from build123d import *

# Parameters (mm, degrees)
SKETCH1_R           = 1.75
SKETCH1_R_2         = 3.175
SKETCH1_R_3         = 1.778
BOSS_EXTRUDE1_DEPTH = 5.461


with BuildPart() as part:
    # Sketch1 → Boss-Extrude1 (new body)
    with BuildSketch(Plane(origin=(0, 0, 0), x_dir=(1, 0, 0), z_dir=(0, 1, 0))):
        with BuildLine():
            Line((-36.075553112, 16.34222836), (-43.713289862, 9.687095487))
            ThreePointArc((-43.713289862, 9.687095487), (-46.071262537, 8.895051227), (-48.298660873, 10.002329828))
            Line((-48.298660873, 10.002329828), (-49.01441114, 10.823757773))
            ThreePointArc((-49.01441114, 10.823757773), (-49.677098428, 12.125807852), (-49.646194202, 13.586469955))
            ThreePointArc((-49.646194202, 13.586469955), (-47.370124011, 20.134748964), (-44.234733225, 26.317772344))
            ThreePointArc((-44.234733225, 26.317772344), (-39.855484626, 29.811728531), (-34.259632886, 29.543416329))
            Line((-34.259632886, 29.543416329), (5.363638877, 12.388760148))
            ThreePointArc((5.363638877, 12.388760148), (7.44200849, -11.263503435), (-13.499793526, -0.074664302))
            Line((-13.499793526, -0.074664302), (-36.075553112, 16.34222836))
        make_face()
        with Locations((8, 0)):
            Circle(SKETCH1_R, mode=Mode.SUBTRACT)
        with Locations((0, -8)):
            Circle(SKETCH1_R, mode=Mode.SUBTRACT)
        with Locations((-8, 0)):
            Circle(SKETCH1_R, mode=Mode.SUBTRACT)
        with Locations((0, 8)):
            Circle(SKETCH1_R, mode=Mode.SUBTRACT)
        Circle(SKETCH1_R_2, mode=Mode.SUBTRACT)
        with Locations((-20.862458922, 15.093717491)):
            Circle(SKETCH1_R_3, mode=Mode.SUBTRACT)
        with Locations((-37.413253893, 22.259284205)):
            Circle(SKETCH1_R_3, mode=Mode.SUBTRACT)
    extrude(amount=BOSS_EXTRUDE1_DEPTH)


solid = part.part
Geometry: final body of the model. Coordinates: model frame, mm. A direction names the side the tool comes from. Give positions to 0.01 mm unless a question says otherwise; leave off trailing zeros. Loops run counter-clockwise (first coordinate to the right, second up) from the corner with the lowest first, then second, coordinate; pieces in that order, holes last. Notation, with made-up numbers: (23, 4.5) - (42, 4.5) arc R10 ccw to (42, 17.5) - close; hole circle Ø4 at (-15.75, -12.75). An arc over 180 degrees is marked (long way). Answer as CSV lines item,"result". Start each with the question number.
1. Draft query along Z for faces 3 (the face through (-39.932, 2.692, -29.787)), 4 (the face through (-0.69, 2.69, 3.1)), 5 (the face through (-18, 5.461, -9)). Return one class per face: released by +Z, released by -Z, zero draft, split by the parting line, or undercut.
2. Section D-D, the plane y = 3.95. Give the number of separate pieces and of enclosed holes in the cut face, plus the area to 3 significant figures.
3. Reachability of faces 1 (the face through (-0.228, 2.692, -9.735)), 2 (the face through (-24.63, 2.69, -8.02)) from +Z, -Z, +X, -X, +Y, -Y: full face, straight path, thin tool, end or side. Return the list, or none.
4. Section C-C, the plane x = 8. Return loops of the section in (y, z).
5. Ray query, L1, parallel to Z at x = 0, y = 2.5 (3 decimals); L2, parallel to X at y = 1.85, z = 0 (3 decimals); L3, parallel to X at y = 4.2, z = 1. Return the intervals inside material, ascending.
6. Pin query (flat end, axial travel): P1, Ø1, axis at y = 1.5, z = -2.5, coming from the +X side; P2, Ø3, axis at x = -20.5, y = 2.5, coming from the +Z side. Return the tip coordinate at first contact, or that it passes through.
7. Section B-B, the plane x = 0. Return loops of the section in (y, z) (3 decimals), plus the area to 3 significant figures.
8. Section A-A, the plane z = -8. Return loops of the section in (x, y), plus the area to 3 significant figures.
Answers:
1,face 3,"released by -Z"
1,face 4,"undercut"
1,face 5,"zero draft"
2,separate pieces,"1"
2,enclosed holes,"7"
2,area,"1,170 mm2"
3,face 1,"+Y, -Y"
3,face 2,"+Z, +Y, -Y"
4,outline,"(0, -10.87) - (5.46, -10.87) - (5.46, -1.75) - (0, -1.75) - close; (0, 1.75) - (5.46, 1.75) - (5.46, 10.87) - (0, 10.87) - close"
5,L1,"z = -14.711 to -9.75, -6.25 to -3.175, 3.175 to 6.25, 9.75 to 13.5"
5,L2,"x = -13.602 to -9.75, -6.25 to -3.175, 3.175 to 6.25, 9.75 to 13.5"
5,L3,"x = -13.46 to -9.44, -6.56 to -3.01, 3.01 to 6.56, 9.44 to 13.46"
6,P1,"stops at x = 13.35"
6,P2,"stops at z = -3.93"
7,outline,"(0, -14.711) - (5.461, -14.711) - (5.461, -9.75) - (0, -9.75) - close; (0, -6.25) - (5.461, -6.25) - (5.461, -3.175) - (0, -3.175) - close; (0, 3.175) - (5.461, 3.175) - (5.461, 6.25) - (0, 6.25) - close; (0, 9.75) - (5.461, 9.75) - (5.461, 13.5) - (0, 13.5) - close"
7,area,"81.2 mm2"
8,outline,"(-24.6, 0) - (-1.75, 0) - (-1.75, 5.46) - (-24.6, 5.46) - close; (1.75, 0) - (10.87, 0) - (10.87, 5.46) - (1.75, 5.46) - close"
8,area,"175 mm2"
